Autodesk Fusion 360 part; units mm, degrees
sketch "Skizze1" plane through (0, 0, 0) normal (0, 0, 1) x (1, 0, 0)
  line L0 (0, 0) -> (20, 0)
  line L1 (20, 0) -> (20, 20)
  line L2 (20, 20) -> (0, 20)
  line L3 (0, 20) -> (0, 0)
  dimension "d1" = 20
  dimension "d2" = 20
extrude "Extrusion1" add sketch "Skizze1" along normal blind 50
extrude "Extrusion2" add 1 faces at (20, 6.6667, 16.6667) along direction (1, 0, 0) blind 20
sketch "Skizze2" plane through (0, 0, 0) normal (0, -1, 0) x (1, 0, 0)
  line L0 (0, 0) -> (40, 0)
  line L1 (40, 0) -> (40, 50)
  line L2 (40, 50) -> (0, 50)
  line L3 (0, 50) -> (0, 0)
  line L4 (0, 50) -> (20, 50)
  line L5 (20, 50) -> (20, 0)
  line L6 (20, 0) -> (0, 0)
  line L7 (0, 0) -> (0, 50)
  dimension "d7" = 20
  dimension "d8" = 50
extrude "Extrusion3" add sketch "Skizze2" along normal blind 20 contours L0 L2 L3 L4 L5 L6 L7
hole "Bohrung1" at (10, 10, 50) direction (0, 0, -1) diameter 5.5 depth 50 tip angle 118
hole "Bohrung2" at (30, 10, 50) direction (0, 0, -1) diameter 5.2 depth 50 tip angle 118 counterbore diameter 10 counterbore depth 40
hole "Bohrung3" at (10, -10, 50) direction (0, 0, -1) diameter 5.2 depth 50 tip angle 180 counterbore diameter 10 counterbore depth 40
extrude "Extrusion4" add 1 faces at (40, 6.6667, 16.6667) along direction (1, 0, 0) blind 10
extrude "Extrusion5" add 1 faces at (6.6667, -20, 16.6667) along direction (0, -1, 0) blind 10
hole "Bohrung4" at (50, 10, 40) direction (-1, 0, 0) diameter 4.7 depth 10 tip angle 180
hole "Bohrung5" at (50, 10, 10) direction (-1, 0, 0) diameter 4.7 depth 10 tip angle 180
hole "Bohrung6" at (10, -30, 40) direction (0, 1, 0) diameter 4.7 depth 10 tip angle 180
hole "Bohrung7" at (10, -30, 10) direction (0, 1, 0) diameter 4.7 depth 10 tip angle 180
extrude "Extrusion6" add 1 faces at (33.3333, 20, 33.3333) along direction (0, 1, 0) blind 5
extrude "Extrusion7" add 1 faces at (0, 6.6667, 33.3333) along direction (-1, 0, 0) blind 5
The model under review builds one solid part; all positions refer to its coordinate system, in mm. A direction names the side the tool comes from. Give positions to 0.01 mm unless a question says otherwise; leave off trailing zeros. Write each loop counter-clockwise with the first axis right and the second up, starting at its lowest first coordinate (ties: lowest second). Pieces come first, ordered by that corner, then holes.
(1) Consider section B-B, the plane z = 40. Give the boundary of the cut face in (x, y).
(2) Consider section C-C, the plane y = -10. Give the boundary of the cut face in (x, z).
(3) Consider section D-D, the plane x = 10. Give the boundary of the cut face in (y, z), and give its area (3 significant figures).
(4) Consider section A-A, the plane x = 30. Give the boundary of the cut face in (y, z), and give its area (3 significant figures).
(5) To check wall thickness, follow L1, parallel to X at y = 10, z = 3; L2, parallel to X at y = 10, z = 23; L3, parallel to Z at x = 10, y = -25.25. State the ranges of each line that lie inside material, in increasing order.
(6) For P1, Ø4, axis at y = 9, z = 9, coming from the +X side; P2, Ø1.4, axis at x = 9, z = 9.5, coming from the -Y side; P3, Ø3, axis at x = 10, y = -10, coming from the -Z side; P4, Ø10, axis at y = -18.5, z = 43, coming from the +X side, all flat-tipped, find the tip position at first contact; note any pin that passes through.
(7) Tool access review of faces 5 (the cylindrical face through (10.9, -24.93, 37.83)), 6 (the flat face through (40, 10, 40)), 7 (the flat face through (32, 8, 10)): name each direction out of +Z, -Z, +X, -X, +Y, -Y from which nothing blocks a thin tool from reaching the whole face with its end or side.
(8) The part is to be moulded in two halves that separate along Y. For faces 1 (the flat face through (20, -15, 25)), 2 (the cylindrical face through (11.05, 7.46, 24.65)), 3 (the flat face through (8, -30, 25)), 4 (the cylindrical face through (8.5, -14.77, 29.72)), say which applies: released by +Y, released by -Y, zero draft, split by the parting line, or undercut.
Returned:
1. outline: (-5, -30) - (7.65, -30) - (7.65, -20) - (12.35, -20) - (12.35, -30) - (20, -30) - (20, 0) - (50, 0) - (50, 7.65) - (40, 7.65) - (40, 12.35) - (50, 12.35) - (50, 25) - (-5, 25) - close; hole circle Ø10 at (10, -10); hole circle Ø5.5 at (10, 10); hole circle Ø10 at (30, 10)
2. outline: (-5, 0) - (7.4, 0) - (7.4, 10) - (5, 10) - (5, 50) - (-5, 50) - close; (12.6, 0) - (20, 0) - (20, 50) - (15, 50) - (15, 10) - (12.6, 10) - close
3. outline: (-30, 0) - (-12.6, 0) - (-12.6, 10) - (-15, 10) - (-15, 50) - (-30, 50) - (-30, 42.35) - (-20, 42.35) - (-20, 37.65) - (-30, 37.65) - (-30, 12.35) - (-20, 12.35) - (-20, 7.65) - (-30, 7.65) - close; (-7.4, 0) - (7.25, 0) - (7.25, 50) - (-5, 50) - (-5, 10) - (-7.4, 10) - close; (12.75, 0) - (25, 0) - (25, 50) - (12.75, 50) - close
3. area: 1,930 mm2
4. outline: (0, 0) - (7.4, 0) - (7.4, 10) - (5, 10) - (5, 50) - (0, 50) - close; (12.6, 0) - (25, 0) - (25, 50) - (15, 50) - (15, 10) - (12.6, 10) - close
4. area: 798 mm2
5. L1: x = -5 to 7.25, 12.75 to 27.4, 32.6 to 50
5. L2: x = -5 to 7.25, 12.75 to 25, 35 to 50
5. L3: z = 0 to 7.65, 12.35 to 37.65, 42.35 to 50
6. P1: stops at x = 50
6. P2: stops at y = -20
6. P3: passes through
6. P4: stops at x = 20
7. face 5: -Y
7. face 6: +X
7. face 7: +Z
8. face 1: zero draft
8. face 2: undercut
8. face 3: released by -Y
8. face 4: undercut
